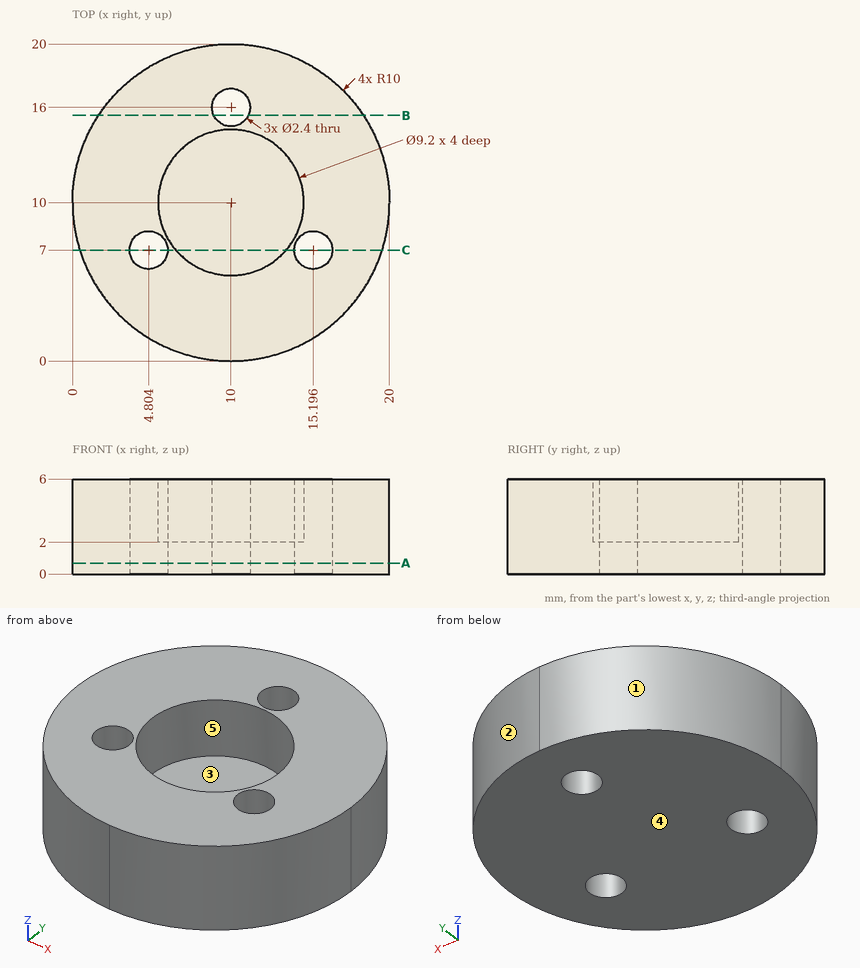
Geometry check sheet. Reference: drawing and pictorial views, mm from the part's lowest x, y, z. A direction names the side the tool comes from. Coordinates: 2 decimals unless noted, no trailing zeros. Order: outer loops, then holes, each group sorted by start corner. A loop starts at its lowest first (then second) coordinate and runs counter-clockwise, first axis right, second up. Notation, with made-up numbers: (51.25, 9) -> (72.25, 9) arc R23 ccw to (72.25, 20) -> close; hole circle Ø9 at (-11.5, 22). An arc over 180 degrees is marked (long way). Use CSV: the item, a comma, the result in double quotes. Start each with the question number.
Q1. Section check A-A, the plane z = 0.7. Give the number of separate pieces and of enclosed holes in the cut face, and give its area (3 significant figures).
Q2. Section check C-C, the plane y = 7. Record the cut outline in (x, z).
Q3. Depth check by flat-ended pin: P1, Ø1, axis at x = 8, z = 2, coming from the +Y side; P2, Ø2, axis at x = 4.8, y = 7, coming from the +Z side; P3, Ø1, axis at y = 3, z = 4, coming from the +X side; P4, Ø3, axis at x = 10, y = 11.5, coming from the +Z side. Enter the tip coordinate at first touch or a pass-through.
Q4. Draft check along X on the marked faces 1, 2 and 3. Enter one of: +X half, -X half, draft (parallel to the pull), parting line (faces both ways), or undercut.
Q5. Tool access check on the marked faces 4 and 5. Record the directions out of +Z, -Z, +X, -X, +Y, -Y that give a thin tool (end or side, any length) a straight path to the whole face; none if there is none.
Q6. Thickness scan on line 1 along Y through (x, z) = (10, 2.4); line 2 along X through (y, z) = (6.5, 1.8) (1 decimal); line 3 along Z through (x, y) = (8.5, 10). Record the ranges inside material, lowest first.
Q7. Section check B-B, the plane y = 15.5. Record the cut outline in (x, z).
Returned:
1,separate pieces,"1"
1,enclosed holes,"3"
1,area,"301 mm^2"
2,outline,"(0.46, 0) -> (3.6, 0) -> (3.6, 6) -> (0.46, 6) -> close; (6, 0) -> (14, 0) -> (14, 6) -> (13.49, 6) -> (13.49, 2) -> (6.51, 2) -> (6.51, 6) -> (6, 6) -> close; (16.4, 0) -> (19.54, 0) -> (19.54, 6) -> (16.4, 6) -> close"
3,P1,"stops at y = 19.89"
3,P2,"passes through"
3,P3,"stops at x = 17.6"
3,P4,"stops at z = 2"
4,face 1,"-X half"
4,face 2,"+X half"
4,face 3,"undercut"
5,face 4,"-Z, +X, -X, +Y, -Y"
5,face 5,"+Z"
6,line 1,"y = 0 to 5.4, 14.6 to 14.8, 17.2 to 20"
6,line 2,"x = 0.6 to 3.7, 5.9 to 14.1, 16.3 to 19.4"
6,line 3,"z = 0 to 2"
7,outline,"(1.65, 0) -> (8.91, 0) -> (8.91, 6) -> (1.65, 6) -> close; (11.09, 0) -> (18.35, 0) -> (18.35, 6) -> (11.09, 6) -> close"
